```python
from build123d import *

# Parameters (mm, degrees)
SKETCH2_W           = 25.4
SKETCH2_H           = 25.4
BOSS_EXTRUDE6_DEPTH = 5
BOSS_EXTRUDE7_DEPTH = 5
FILLET1_R           = 5
SKETCH5_R           = 1
CUT_EXTRUDE1_DEPTH  = 5
SKETCH6_W           = 28.098270468
SKETCH6_H           = 9.80175879
CUT_EXTRUDE2_DEPTH  = 49.905214446
SKETCH7_W           = 43.4
SKETCH7_H           = 25.4
SKETCH7_R           = 2.5
BOSS_EXTRUDE8_DEPTH = 5
SKETCH8_R           = 2.5
CUT_EXTRUDE3_DEPTH  = 10


with BuildPart() as part:
    # Sketch2 → Boss-Extrude6 (new body)
    with BuildSketch(Plane(origin=(0, 0, 0), x_dir=(1, 0, 0), z_dir=(0, 1, 0))):
        with Locations((12.7, 12.7)):
            Rectangle(SKETCH2_W, SKETCH2_H)
    extrude(amount=BOSS_EXTRUDE6_DEPTH)

    # Sketch4 → Boss-Extrude7 (add)
    with BuildSketch(Plane.XZ):
        with BuildLine():
            Line((25.4, 0), (25.4, -9.7))
            ThreePointArc((25.4, -9.7), (34.4, -12.7), (25.4, -15.7))
            Line((25.4, -15.7), (25.4, -25.4))
            Line((25.4, -25.4), (15.7, -25.4))
            ThreePointArc((15.7, -25.4), (12.7, -34.4), (9.7, -25.4))
            Line((9.7, -25.4), (0, -25.4))
            Line((0, -25.4), (0, -15.7))
            ThreePointArc((0, -15.7), (-9, -12.7), (0, -9.7))
            Line((0, -9.7), (0, 0))
            Line((0, 0), (9.7, 0))
            Line((9.7, 0), (15.7, 0))
            Line((15.7, 0), (25.4, 0))
        make_face()
    extrude(amount=-BOSS_EXTRUDE7_DEPTH)

    # Fillet1
    fillet1_edges = [part.edges().sort_by_distance(p)[0] for p in [
        (25.4, 2.5, -9.7),
        (25.4, 2.5, -15.7),
        (15.7, 2.5, -25.4),
        (9.7, 2.5, -25.4),
        (0, 2.5, -15.7),
        (0, 2.5, -9.7),
    ]]
    fillet(fillet1_edges, radius=FILLET1_R)

    # Sketch5 → Cut-Extrude1 (cut)
    with BuildSketch(Plane(origin=(0, 5, 0), x_dir=(1, 0, 0), z_dir=(0, 1, 0))):
        with Locations(Location((-4, 12.7, 0), (0, 0, 270))):
            Circle(SKETCH5_R)
        with Locations(Location((12.7, 29.4, 0), (0, 0, 270))):
            Circle(SKETCH5_R)
        with Locations(Location((29.4, 12.7, 0), (0, 0, 270))):
            Circle(SKETCH5_R)
    extrude(amount=-CUT_EXTRUDE1_DEPTH, mode=Mode.SUBTRACT)

    # Sketch6 → Cut-Extrude2 (cut, through all)
    with BuildSketch(Plane(origin=(0, 5, 0), x_dir=(1, 0, 0), z_dir=(0, 1, 0))):
        with Locations((14.049135234, 30.300879395)):
            Rectangle(SKETCH6_W, SKETCH6_H)
    extrude(amount=-CUT_EXTRUDE2_DEPTH, mode=Mode.SUBTRACT)

    # Sketch7 → Boss-Extrude8 (add)
    with BuildSketch(Plane(origin=(0, 5, 0), x_dir=(1, 0, 0), z_dir=(0, 1, 0))):
        with Locations((12.7, 12.7)):
            Rectangle(SKETCH7_W, SKETCH7_H)
        with Locations((-4, 12.7)):
            Circle(SKETCH7_R, mode=Mode.SUBTRACT)
        with Locations((29.4, 12.7)):
            Circle(SKETCH7_R, mode=Mode.SUBTRACT)
    extrude(amount=-BOSS_EXTRUDE8_DEPTH)

    # Sketch8 → Cut-Extrude3 (cut)
    with BuildSketch(Plane(origin=(0, 5, 0), x_dir=(1, 0, 0), z_dir=(0, 1, 0))):
        with Locations(Location((-4, 12.7, 0), (0, 0, 270))):
            Circle(SKETCH8_R)
        with Locations(Location((29.4, 12.7, 0), (0, 0, 270))):
            Circle(SKETCH8_R)
    extrude(amount=-CUT_EXTRUDE3_DEPTH, mode=Mode.SUBTRACT)


solid = part.part
```
The model under review builds one solid part; all positions refer to its coordinate system, in mm. Give positions to 0.01 mm unless a question says otherwise; leave off trailing zeros. Write each loop counter-clockwise with the first axis right and the second up, starting at its lowest first coordinate (ties: lowest second). Pieces come first, ordered by that corner, then holes. Notation, with made-up numbers: M 55.25,63 L 61.25,63 A20 ccw 61.25,79 Z; hole C 53.5,19.25 d1. An arc over 180 degrees is marked long. Write each question's results on one line, items separated by ' | '. Start each with the question number.
1. We need section A-A (z = -12.7). Write out the cut boundary in (x, y), and give its area (3 significant figures).
2. We need section C-C (y = 4.25). Write out the cut boundary in (x, z), and give its area (3 significant figures).
3. Mouldability with a two-part tool opening along X and no side actions: class faces 1 (the flat face through (34.4, 3, -13)), 2 (the cylindrical face through (31.88, 2.54, -13.03)), 3 (the flat face through (-9, 3, -13)), 4 (the flat face through (12, 3, -25.4)) as released by +X, released by -X, zero draft, split by the parting line, or undercut.
4. We need section D-D (x = -5). Write out the cut boundary in (y, z), and give its area (3 significant figures).
5. For probe 1 along X at (y, z) = (3.75, -12.75); probe 2 along X at (y, z) = (4.55, -15); probe 3 along Z at (x, y) = (30, 0.55), list the stretches that pass through material, from the lowest coordinate up. Write a range as [from, to].
6. We need section B-B (x = 29.4). Write out the cut boundary in (y, z), and give its area (3 significant figures).
Results found:
1) outline: M -9,0 L -6.5,0 L -6.5,5 L -9,5 Z; M -1.5,0 L 26.9,0 L 26.9,5 L -1.5,5 Z; M 31.9,0 L 34.4,0 L 34.4,5 L 31.9,5 Z | area: 167 mm^2
2) outline: M -9,-25.4 L 34.4,-25.4 L 34.4,0 L -9,0 Z; hole C -4,-12.7 d5; hole C 29.4,-12.7 d5 | area: 1,060 mm^2
3) face 1: released by +X | face 2: undercut | face 3: released by -X | face 4: zero draft
4) outline: M 0,-25.4 L 5,-25.4 L 5,-14.99 L 0,-14.99 Z; M 0,-10.41 L 5,-10.41 L 5,0 L 0,0 Z | area: 104 mm^2
5) probe 1: x = [-9, -6.5], [-1.5, 26.9], [31.9, 34.4] | probe 2: x = [-9, -4.98], [-3.02, 28.42], [30.38, 34.4] | probe 3: z = [-25.4, -15.13], [-10.27, 0]
6) outline: M 0,-25.4 L 5,-25.4 L 5,-15.2 L 0,-15.2 Z; M 0,-10.2 L 5,-10.2 L 5,0 L 0,0 Z | area: 102 mm^2
